from build123d import *

# Parameters (mm, degrees)
SKETCH1_W           = 120
SKETCH1_H           = 80
BOSS_EXTRUDE1_DEPTH = 15
SKETCH2_R           = 40
BOSS_EXTRUDE2_DEPTH = 20
SKETCH3_R           = 30
CUT_EXTRUDE3_DEPTH  = 15
SKETCH4_R           = 15
CUT_EXTRUDE4_DEPTH  = 29
BOSS_EXTRUDE5_DEPTH = 20
SKETCH8_R           = 16
CUT_EXTRUDE6_DEPTH  = 20


with BuildPart() as part:
    # Sketch1 → Boss-Extrude1 (new body)
    with BuildSketch(Plane(origin=(0, 0, 0), x_dir=(1, 0, 0), z_dir=(0, 1, 0))):
        Rectangle(SKETCH1_W, SKETCH1_H)
    extrude(amount=BOSS_EXTRUDE1_DEPTH)

    # Sketch2 → Boss-Extrude2 (add)
    with BuildSketch(Plane(origin=(0, 15, 0), x_dir=(1, 0, 0), z_dir=(0, 1, 0))):
        with Locations(Location((0, 0, 0), (0, 0, 270))):
            Circle(SKETCH2_R)
    extrude(amount=BOSS_EXTRUDE2_DEPTH)

    # Sketch3 → Cut-Extrude3 (cut)
    with BuildSketch(Plane(origin=(0, 35, 0), x_dir=(1, 0, 0), z_dir=(0, 1, 0))):
        with Locations(Location((0, 0, 0), (0, 0, 270))):
            Circle(SKETCH3_R)
    extrude(amount=-CUT_EXTRUDE3_DEPTH, mode=Mode.SUBTRACT)

    # Sketch4 → Cut-Extrude4 (cut)
    with BuildSketch(Plane(origin=(0, 20, 0), x_dir=(1, 0, 0), z_dir=(0, 1, 0))):
        with Locations(Location((0, 0, 0), (0, 0, 270))):
            Circle(SKETCH4_R)
    extrude(amount=-CUT_EXTRUDE4_DEPTH, mode=Mode.SUBTRACT)

    # Sketch5 → Boss-Extrude5 (add)
    with BuildSketch(Plane(origin=(60, 0, 0), x_dir=(0, 0, -1), z_dir=(1, 0, 0))):
        with BuildLine():
            Line((-40, 0), (40, 0))
            Line((40, 0), (40, -50))
            ThreePointArc((40, -50), (0, -90), (-40, -50))
            Line((-40, -50), (-40, 0))
        make_face()
    boss_extrude5 = extrude(amount=-BOSS_EXTRUDE5_DEPTH)

    # Sketch8 → Cut-Extrude6 (cut)
    with BuildSketch(Plane(origin=(60, 0, 0), x_dir=(0, 0, -1), z_dir=(1, 0, 0))):
        with Locations((0, -50)):
            Circle(SKETCH8_R)
    cut_extrude6 = extrude(amount=-CUT_EXTRUDE6_DEPTH, mode=Mode.SUBTRACT)

    # Mirror1: Boss-Extrude5, Cut-Extrude6 across plane
    add(boss_extrude5.mirror(Plane(origin=(0, 0, 0), x_dir=(0, 0, 1), z_dir=(1, 0, 0))))
    add(cut_extrude6.mirror(Plane(origin=(0, 0, 0), x_dir=(0, 0, 1), z_dir=(1, 0, 0))), mode=Mode.SUBTRACT)


solid = part.part
Geometry: final body of the model. Coordinates: model frame, mm. A direction names the side the tool comes from. Coordinates: 2 decimals unless noted, no trailing zeros. Order: outer loops, then holes, each group sorted by start corner. A loop starts at its lowest first (then second) coordinate and runs counter-clockwise, first axis right, second up.
(1) Section query C-C (x = -48.5). Return the cut outline in (y, z), plus the area to 3 significant figures.
(2) Draft query along X for faces 1 (the face through (-40, -34, -9)), 2 (the face through (60, -25, -1)), 3 (the face through (0.66, 10.14, -14.985)), 4 (the face through (50.14, -89.99, -0.88)). Return one class per face: pulls with the +X half, pulls with the -X half, needs draft (parallel to the pull), parting line crosses it, or undercut.
(3) Access query for faces 5 (the face through (-14, 5, -40)), 6 (the face through (1.32, 27.6, -29.97)), 7 (the face through (40, -34, -9)), 8 (the face through (43, 15, -1)), 9 (the face through (-44, 15, -1)). Directions: +Z, -Z, +X, -X, +Y, -Y. A direction counts if a zero-diameter tool reaches every point of the face in a straight line with its end or side. Return the directions, or none.
(4) Section query D-D (z = 28). Return the cut outline in (x, y).
(5) Material intervals for probe 1 along Y at (x, z) = (-54, 0); probe 2 along X at (y, z) = (-34, 26); probe 3 along X at (y, z) = (5.5, 0), sorted ascending.
(6) Section query B-B (y = 6.5). Return the cut outline in (x, z), plus the area to 3 significant figures.
(7) Section query A-A (z = 0). Return the cut outline in (x, y).
(8) First-contact query: pin 1 (1 mm diameter, centred on x = 12.5, z = 15.5, fed in from +Y); pin 2 (2 mm diameter, centred on x = 34.5, z = 11.5, fed in from -Y). Flat tips, straight axial feed; report the tip coordinate or a pass-through.
Solution:
1. outline: (-50, -40) - (15, -40) - (15, 40) - (-50, 40) arc R40 ccw to start; hole circle Ø32 at (-50, 0)
1. area: 6,910 mm2
2. face 1: undercut
2. face 2: pulls with the +X half
2. face 3: undercut
2. face 4: needs draft
3. face 5: -Z, +X, -X, +Y, -Y
3. face 6: +Y
3. face 7: +Z, -Z, -Y
3. face 8: +X, +Y
3. face 9: -X, +Y
4. outline: (-60, -78.57) - (-40, -78.57) - (-40, 0) - (40, 0) - (40, -78.57) - (60, -78.57) - (60, 15) - (28.57, 15) - (28.57, 35) - (10.77, 35) - (10.77, 20) - (-10.77, 20) - (-10.77, 35) - (-28.57, 35) - (-28.57, 15) - (-60, 15) - close
5. probe 1: y = -90 to -66, -34 to 15
5. probe 2: x = -60 to -40, 40 to 60
5. probe 3: x = -60 to -15, 15 to 60
6. outline: (-60, -40) - (60, -40) - (60, 40) - (-60, 40) - close; hole circle Ø30 at (0, 0)
6. area: 8,890 mm2
7. outline: (-60, -90) - (-40, -90) - (-40, -66) - (-60, -66) - close; (-60, -34) - (-40, -34) - (-40, 0) - (-15, 0) - (-15, 20) - (-30, 20) - (-30, 35) - (-40, 35) - (-40, 15) - (-60, 15) - close; (15, 0) - (40, 0) - (40, -34) - (60, -34) - (60, 15) - (40, 15) - (40, 35) - (30, 35) - (30, 20) - (15, 20) - close; (40, -90) - (60, -90) - (60, -66) - (40, -66) - close
8. pin 1: stops at y = 20
8. pin 2: stops at y = 0
